Source: CAD feature listing. Evaluate the final solid. Frame: model axes, mm. Round coordinates to 2 decimals unless told otherwise and drop trailing zeros. Loops run counter-clockwise (first coordinate to the right, second up) from the corner with the lowest first, then second, coordinate; pieces in that order, holes last. Notation, with made-up numbers: (9, 79) -> (47, 79) arc R18 ccw to (47, 113) -> close; hole circle Ø3 at (25.25, 28). An arc over 180 degrees is marked (long way). Put each result on its own line as item: value. Start each with the question number.
1. Draft query along X for faces 1 (the flat face through (0, 0, 0)), 2 (the flat face through (-3, 0, 6)), 3 (the cylindrical face through (9.8, 0.25, 3.7)). Return one class per face: pulls with the +X half, pulls with the -X half, needs draft (parallel to the pull), parting line crosses it, or undercut.
2. Material intervals for L1, parallel to X at y = -3, z = 0; L2, parallel to Y at x = -10.5, z = 0.75; L3, parallel to Z at x = 3.5, y = -3.75, sorted ascending.
3. Cut plane A-A (y = 3). Return the cut outline in (x, z).
4. Contact query for flat-ended pins moving along their axis: pin 1 (1.5 mm diameter, centred on x = -4, y = -4, fed in from -Z); pin 2 (12 mm diameter, centred on x = 5.5, z = 9.5, fed in from +Y); pin 3 (5 mm diameter, centred on x = 11, y = 4.5, fed in from +Z); pin 4 (4 mm diameter, centred on x = 9.5, y = 3.5, fed in from +Z). Output: stop coordinate, or through.
```python
from build123d import *

# Parameters (mm, degrees)
EXTRUDE1_DEPTH = 6.35
EXTRUDE1_TAPER = 7.000000000000015
FILLET1_R      = 2.2224999999999997
SKETCH2_R      = 6.35
SKETCH2_R_2    = 4.7625
EXTRUDE2_DEPTH = 6.35
FILLET2_R      = 0.762


with BuildPart() as part:
    # Sketch1 → Extrude1 (new body)
    with BuildSketch(Plane(origin=(0, 0, 0), x_dir=(1, 0, 0), z_dir=(0, 1, 0))):
        with BuildLine():
            ThreePointArc((3.174999999999997, 12.7), (2.4e-15, 15.092534109076349), (-3.17499999999998, 12.7))
            Line((-3.17499999999998, 12.7), (-4.812500349494196, 6.989357629379411))
            ThreePointArc((-4.812500349494196, 6.989357629379411), (-5.619442203831074, 5.619442203831092), (-6.989357629379396, 4.812500349494221))
            Line((-6.989357629379396, 4.812500349494221), (-12.699999999999969, 3.1750000000000442))
            ThreePointArc((-12.699999999999969, 3.1750000000000442), (-15.092534109076396, -4e-16), (-12.699999999999969, -3.1750000000000442))
            Line((-12.699999999999969, -3.1750000000000442), (-6.989357629379396, -4.812500349494221))
            ThreePointArc((-6.989357629379396, -4.812500349494221), (-5.619442203831074, -5.619442203831092), (-4.812500349494196, -6.989357629379411))
            Line((-4.812500349494196, -6.989357629379411), (-3.17499999999998, -12.7))
            ThreePointArc((-3.17499999999998, -12.7), (3.14e-15, -15.092534109076366), (3.174999999999997, -12.7))
            Line((3.174999999999997, -12.7), (4.812500349494196, -6.989357629379411))
            ThreePointArc((4.812500349494196, -6.989357629379411), (5.619442203831074, -5.619442203831092), (6.989357629379396, -4.812500349494221))
            Line((6.989357629379396, -4.812500349494221), (12.699999999999985, -3.1750000000000442))
            ThreePointArc((12.699999999999985, -3.1750000000000442), (15.0925341090764, 0), (12.699999999999985, 3.1750000000000442))
            Line((12.699999999999985, 3.1750000000000442), (6.989357629379396, 4.812500349494221))
            ThreePointArc((6.989357629379396, 4.812500349494221), (5.619442203831074, 5.619442203831092), (4.812500349494196, 6.989357629379411))
            Line((4.812500349494196, 6.989357629379411), (3.174999999999997, 12.7))
        make_face()
    extrude(amount=EXTRUDE1_DEPTH, taper=EXTRUDE1_TAPER)

    # Fillet1
    fillet1_edges = [part.edges().sort_by_distance(p)[0] for p in [
        (3.2442717699186887, 6.35, 9.629769340379289),
        (5.068123801520522, 6.35, 5.068123801520543),
        (9.629769340379273, 6.35, 3.244271769918725),
        (14.312852147342955, 6.35, 1.33e-15),
        (9.629769340379273, 6.35, -3.2442717699187247),
        (5.068123801520526, 6.35, -5.06812380152054),
        (3.2442717699186923, 6.35, -9.629769340379278),
        (1.443e-14, 6.35, -14.312852147342902),
        (-3.2442717699186843, 6.35, -9.629769340379275),
        (-5.068123801520527, 6.35, -5.068123801520538),
        (-9.629769340379273, 6.35, -3.244271769918723),
        (-14.31285214734295, 6.35, 2.2e-16),
        (-9.629769340379273, 6.35, 3.244271769918723),
        (-5.068123801520526, 6.35, 5.06812380152054),
        (-3.2442717699186803, 6.35, 9.629769340379287),
        (1.155e-14, 6.35, 14.312852147342921),
    ]]
    fillet(fillet1_edges, radius=FILLET1_R)

    # Sketch2 → Extrude2 (add)
    with BuildSketch(Plane.XZ):
        with Locations(Location((0, 0, 0), (0, 0, 270))):
            Circle(SKETCH2_R)
        with Locations(Location((0, 0, 0), (0, 0, 270))):
            Circle(SKETCH2_R_2, mode=Mode.SUBTRACT)
    extrude(amount=EXTRUDE2_DEPTH)

    # Fillet2
    fillet2_edges = [part.edges().sort_by_distance(p)[0] for p in [
        (3.9937501747470967, 0, 9.844678814689704),
        (5.619442203831073, 0, 5.619442203831092),
        (7.99e-15, 0, 15.092534109076366),
        (-3.993750174747088, 0, 9.844678814689704),
        (9.84467881468969, 0, 3.9937501747471327),
        (-5.619442203831074, 0, 5.619442203831092),
        (15.0925341090764, 0, 3.3e-16),
        (-9.844678814689683, 0, 3.9937501747471327),
        (9.84467881468969, 0, -3.9937501747471327),
        (-15.092534109076396, 0, -3.3e-16),
        (5.619442203831074, 0, -5.619442203831092),
        (-9.844678814689683, 0, -3.9937501747471327),
        (3.9937501747470967, 0, -9.844678814689704),
        (-5.619442203831073, 0, -5.619442203831092),
        (8.88e-15, 0, -15.092534109076349),
        (-3.9937501747470883, 0, -9.844678814689704),
    ]]
    fillet(fillet2_edges, radius=FILLET2_R)


solid = part.part
```
Solution:
1. face 1: undercut
1. face 2: needs draft
1. face 3: pulls with the +X half
2. L1: x = -6.35 to -4.76, 4.76 to 6.35
2. L2: y = 0 to 6.35
2. L3: z = -5.3 to -3.23, 3.23 to 5.3
3. outline: (-12.6, -2.82) -> (-6.89, -4.46) arc R3.54 cw to (-4.46, -6.89) -> (-2.82, -12.6) arc R2.93 ccw to (2.82, -12.6) -> (4.46, -6.89) arc R3.54 cw to (6.89, -4.46) -> (12.6, -2.82) arc R2.93 ccw to (12.6, 2.82) -> (6.89, 4.46) arc R3.54 cw to (4.46, 6.89) -> (2.82, 12.6) arc R2.93 ccw to (-2.82, 12.6) -> (-4.46, 6.89) arc R3.54 cw to (-6.89, 4.46) -> (-12.6, 2.82) arc R2.93 ccw to start
4. pin 1: stops at z = -5.46
4. pin 2: stops at y = 6.35
4. pin 3: stops at z = 3.87
4. pin 4: stops at z = 4.27
